from build123d import *

# Parameters (mm, degrees)
SKETCH1_R           = 22.5
SKETCH1_R_2         = 11
SKETCH1_R_3         = 1.25
SKETCH1_R_4         = 1.5
BOSS_EXTRUDE1_DEPTH = 6
MOVE_FACE1_BY       = 0.08
MOVE_FACE1_2_BY     = 0.08
MOVE_FACE1_3_BY     = 0.08
MOVE_FACE1_4_BY     = 0.08
MOVE_FACE1_5_BY     = 0.08
MOVE_FACE1_6_BY     = 0.08
MOVE_FACE1_7_BY     = 0.08
MOVE_FACE1_8_BY     = 0.08
MOVE_FACE1_9_BY     = 0.08
MOVE_FACE1_10_BY    = 0.08


with BuildPart() as part:
    # Sketch1 → Boss-Extrude1 (new body)
    with BuildSketch(Plane.XY):
        Circle(SKETCH1_R)
        Circle(SKETCH1_R_2, mode=Mode.SUBTRACT)
        with Locations((0, 15)):
            Circle(SKETCH1_R_3, mode=Mode.SUBTRACT)
        with Locations((10.606601718, 10.606601718)):
            Circle(SKETCH1_R_4, mode=Mode.SUBTRACT)
        with Locations((15, 0)):
            Circle(SKETCH1_R_3, mode=Mode.SUBTRACT)
        with Locations((10.606601718, -10.606601718)):
            Circle(SKETCH1_R_4, mode=Mode.SUBTRACT)
        with Locations((0, -15)):
            Circle(SKETCH1_R_3, mode=Mode.SUBTRACT)
        with Locations((-10.606601718, -10.606601718)):
            Circle(SKETCH1_R_4, mode=Mode.SUBTRACT)
        with Locations((-15, 0)):
            Circle(SKETCH1_R_3, mode=Mode.SUBTRACT)
        with Locations((-10.606601718, 10.606601718)):
            Circle(SKETCH1_R_4, mode=Mode.SUBTRACT)
    extrude(amount=BOSS_EXTRUDE1_DEPTH)

    # Move Face1: a curved face moved outward by 0.08
    add(Solid.thicken(part.faces().sort_by_distance((-11, 0, 3))[0], MOVE_FACE1_BY))

    # Move Face1 2: a curved face moved outward by 0.08
    add(Solid.thicken(part.faces().sort_by_distance((-22.5, 0, 3))[0], MOVE_FACE1_2_BY))

    # Move Face1 3: a curved face moved outward by 0.08
    add(Solid.thicken(part.faces().sort_by_distance((-1.25, 15, 3))[0], MOVE_FACE1_3_BY))

    # Move Face1 4: a curved face moved outward by 0.08
    add(Solid.thicken(part.faces().sort_by_distance((9.106601718, 10.606601718, 3))[0], MOVE_FACE1_4_BY))

    # Move Face1 5: a curved face moved outward by 0.08
    add(Solid.thicken(part.faces().sort_by_distance((13.75, 0, 3))[0], MOVE_FACE1_5_BY))

    # Move Face1 6: a curved face moved outward by 0.08
    add(Solid.thicken(part.faces().sort_by_distance((9.106601718, -10.606601718, 3))[0], MOVE_FACE1_6_BY))

    # Move Face1 7: a curved face moved outward by 0.08
    add(Solid.thicken(part.faces().sort_by_distance((-1.25, -15, 3))[0], MOVE_FACE1_7_BY))

    # Move Face1 8: a curved face moved outward by 0.08
    add(Solid.thicken(part.faces().sort_by_distance((-12.106601718, -10.606601718, 3))[0], MOVE_FACE1_8_BY))

    # Move Face1 9: a curved face moved outward by 0.08
    add(Solid.thicken(part.faces().sort_by_distance((-16.25, 0, 3))[0], MOVE_FACE1_9_BY))

    # Move Face1 10: a curved face moved outward by 0.08
    add(Solid.thicken(part.faces().sort_by_distance((-12.106601718, 10.606601718, 3))[0], MOVE_FACE1_10_BY))


solid = part.part
Here's how the part is built. I have some questions about the finished solid (model axes, mm). Round coordinates to 2 decimals unless told otherwise and drop trailing zeros. Order: outer loops, then holes, each group sorted by start corner. A loop starts at its lowest first (then second) coordinate and runs counter-clockwise, first axis right, second up. Notation, with made-up numbers: M 21,3.25 L 80,3.25 A19 ccw 80,13.25 Z; hole C 3,30.25 d11. An arc over 180 degrees is marked long. Return JSON: item names as keys, results as strings. Group by question number.
1. I'm going to push flat-ended pins straight in: pin 1 Ø3 at (x, z) = (9.5, 3.5) entering from -Y; pin 2 Ø6 at (x, y) = (-16.5, -16) entering from -Z; pin 3 Ø2 at (y, z) = (16.5, 1) entering from +X; pin 4 Ø1 at (x, z) = (6.5, 3.5) entering from -Y. Where does each tip first touch, or does it pass through?
2. If we section it at B-B on y = -15: List the corners of the cut face in (x, z) for me.
3. If we section it at C-C on x = 7: List the corners of the cut face in (y, z) for me, then the cut area to 3 significant figures.
4. If we section it at A-A on x = 0: List the corners of the cut face in (y, z) for me, then the cut area to 3 significant figures.
5. Please list where these lines run through material, in increasing order: probe 1 along Y at (x, z) = (0, 2.5); probe 2 along Y at (x, z) = (-11, 3.45); probe 3 along X at (y, z) = (-10, 0.3).
6. If we mould it in two halves opening along X, with no side actions, what happens to faces 1 (the face through (-10.91, 9.22, 2.96)), 2 (the face through (-4.895, -22.043, 2.958)), 3 (the face through (-5, -10, 0))? For each: pulls with the +X half, pulls with the -X half, needs draft (parallel to the pull), parting line crosses it, or undercut.
Reply:
{
 "1": {"pin 1": "y = -21.12", "pin 2": "z = 0", "pin 3": "x = 16.42", "pin 4": "y = -21.77"},
 "2": {"outline": "M -16.88,0 L -1.17,0 L -1.17,6 L -16.88,6 Z; M 1.17,0 L 16.88,0 L 16.88,6 L 1.17,6 Z"},
 "3": {"outline": "M -21.47,0 L -8.38,0 L -8.38,6 L -21.47,6 Z; M 8.38,0 L 21.47,0 L 21.47,6 L 8.38,6 Z", "area": "157 mm^2"},
 "4": {"outline": "M -22.58,0 L -16.17,0 L -16.17,6 L -22.58,6 Z; M -13.83,0 L -10.92,0 L -10.92,6 L -13.83,6 Z; M 10.92,0 L 13.83,0 L 13.83,6 L 10.92,6 Z; M 16.17,0 L 22.58,0 L 22.58,6 L 16.17,6 Z", "area": "112 mm^2"},
 "5": {"probe 1": "-22.58 to -16.17, -13.83 to -10.92, 10.92 to 13.83, 16.17 to 22.58", "probe 2": "-19.72 to -11.97, -9.24 to 9.24, 11.97 to 19.72", "probe 3": "-20.24 to -11.89, -9.32 to -4.39, 4.39 to 9.32, 11.89 to 20.24"},
 "6": {"face 1": "undercut", "face 2": "parting line crosses it", "face 3": "needs draft"}
}
